Autodesk Inventor part; units mm, degrees
ref_plane "YZ Plane" through (0, 0, 0) normal (1, 0, 0) x (0, 1, 0)
ref_plane "XZ Plane" through (0, 0, 0) normal (0, 1, 0) x (-1, 0, 0)
ref_plane "XY Plane" through (0, 0, 0) normal (0, 0, 1) x (1, 0, 0)
sketch "Szkic1" plane through (0, 0, 0) normal (0, 0, 1) x (1, 0, 0)
  circle A0 centre (0, 0) radius 5.25
  dimension "d0" = 10.5
extrude "Wyciągnięcie proste1" add sketch "Szkic1" along normal blind 5.5
sketch "Szkic2" plane through (0, 0, 5.5) normal (0, 0, 1) x (1, 0, 0)
  circle A0 centre (0, 0) radius 5.25
  circle A1 centre (0, 0) radius 5.85
  dimension "d3" = 11.7
extrude "Wyciągnięcie proste2" add sketch "Szkic2" along normal blind 40 contours A0 | A1
sketch "Szkic3" plane through (0, 0, 45.5) normal (0, 0, 1) x (1, 0, 0)
  circle A0 centre (0, 0) radius 5.85
  circle A1 centre (0, 0) radius 5.55
  dimension "d6" = 11.1
extrude "Wyciągnięcie proste3" add sketch "Szkic3" along normal blind 14.5 contours A1
thread "Gwint1"
sketch "Szkic4" plane through (0, 0, 60) normal (0, 0, 1) x (1, 0, 0)
  circle A0 centre (0, 0) radius 5.25
  dimension "d11" = 10.5
extrude "Wyciągnięcie proste4" add sketch "Szkic4" along normal blind 1
sketch "Szkic5" plane through (0, 0, 61) normal (0, 0, 1) x (1, 0, 0)
  circle A0 centre (0, 0) radius 5.25
  circle A1 centre (-2.2069, 0) radius 2.85
  dimension "d14" = 5.7
extrude "Wyciągnięcie proste5" add sketch "Szkic5" along normal blind 5 contours A1
sketch "Szkic6" plane through (-2.2069, 0, 66) normal (0, 0, 1) x (1, 0, 0)
  circle A0 centre (0, 0) radius 2.85
  circle A1 centre (0, 0) radius 1.8
  point P0 (2.2069, 0)
  dimension "d17" = 3.6
extrude "Wyciągnięcie proste6" add sketch "Szkic6" along normal blind 6 contours A1
properties part number "COTS_GENERIC_Induction_Distance_Sensor"
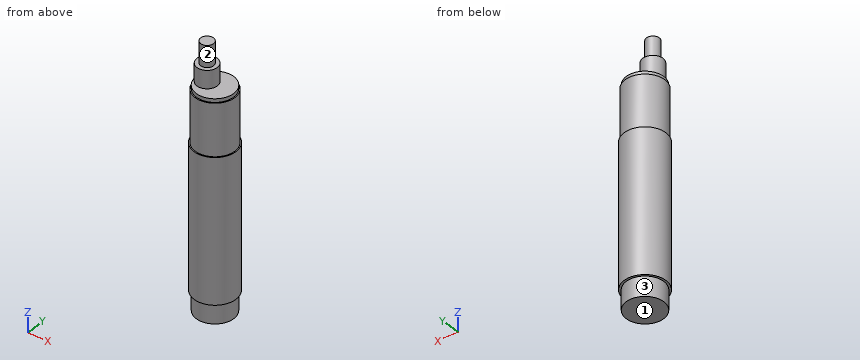
Geometry check sheet. Reference: the model listing, model coordinates, mm. Face numbers are marked on the shaded views. A direction names the side the tool comes from. Round coordinates to 2 decimals unless told otherwise and drop trailing zeros. Order: outer loops, then holes, each group sorted by start corner. A loop starts at its lowest first (then second) coordinate and runs counter-clockwise, first axis right, second up. Notation, with made-up numbers: (-10, 20.25) -> (34, 20.25) arc R21 ccw to (34, 59.25) -> close; hole circle Ø7 at (56.5, 69.25). An arc over 180 degrees is marked (long way). Return JSON: item names as keys, results as strings. Group by question number.
Q1. Section check B-B, the plane x = 4. Record the boundary of the cut face in (y, z), plus the area to 3 significant figures.
Q2. Material ranges on probe 1 along Z at (x, y) = (1.5, 5); probe 2 along Z at (x, y) = (-4, -2); probe 3 along Y at (x, z) = (-0.25, 16.5), recorded low to high. Write a range as from..to.
Q3. Section check D-D, the plane y = 4.5. Record the boundary of the cut face in (x, z).
Q4. Section check A-A, the plane y = 0. Record the boundary of the cut face in (x, z), plus the area to 3 significant figures.
Q5. Gauge pin test, flat ends, axial feed: pin 1 (1 mm diameter, centred on x = -1.5, z = 62.5, fed in from +Y); pin 2 (4 mm diameter, centred on x = 0, z = 54, fed in from +Y); pin 3 (4 mm diameter, centred on x = 4, y = -1.5, fed in from +Z). Record the tip position at first contact, or that the pin passes through.
Q6. Section check C-C, the plane z = 58. Record the boundary of the cut face in (x, y).
Q7. Tool access check on the marked faces 1, 2 and 3. Record the directions out of +Z, -Z, +X, -X, +Y, -Y that give a thin tool (end or side, any length) a straight path to the whole face; none if there is none.
Numbers:
{
 "1": {"outline": "(-4.27, 5.5) -> (-3.4, 5.5) -> (-3.4, 0) -> (3.4, 0) -> (3.4, 5.5) -> (4.27, 5.5) -> (4.27, 45.5) -> (3.85, 45.5) -> (3.85, 60) -> (3.4, 60) -> (3.4, 61) -> (-3.4, 61) -> (-3.4, 60) -> (-3.85, 60) -> (-3.85, 45.5) -> (-4.27, 45.5) -> close", "area": "497 mm^2"},
 "2": {"probe 1": "0..61", "probe 2": "0..66", "probe 3": "-5.84..5.84"},
 "3": {"outline": "(-3.74, 5.5) -> (-2.7, 5.5) -> (-2.7, 0) -> (2.7, 0) -> (2.7, 5.5) -> (3.74, 5.5) -> (3.74, 45.5) -> (3.25, 45.5) -> (3.25, 60) -> (2.7, 60) -> (2.7, 61) -> (-2.7, 61) -> (-2.7, 60) -> (-3.25, 60) -> (-3.25, 45.5) -> (-3.74, 45.5) -> close"},
 "4": {"outline": "(-5.85, 5.5) -> (-5.25, 5.5) -> (-5.25, 0) -> (5.25, 0) -> (5.25, 5.5) -> (5.85, 5.5) -> (5.85, 45.5) -> (5.55, 45.5) -> (5.55, 60) -> (5.25, 60) -> (5.25, 61) -> (0.64, 61) -> (0.64, 66) -> (-0.41, 66) -> (-0.41, 72) -> (-4.01, 72) -> (-4.01, 66) -> (-5.06, 66) -> (-5.06, 61) -> (-5.25, 61) -> (-5.25, 60) -> (-5.55, 60) -> (-5.55, 45.5) -> (-5.85, 45.5) -> close", "area": "747 mm^2"},
 "5": {"pin 1": "y = 2.84", "pin 2": "y = 5.55", "pin 3": "z = 61"},
 "6": {"outline": "circle Ø11.1 at (0, 0)"},
 "7": {"face 1": "-Z, +X, -X, +Y, -Y", "face 2": "+Z", "face 3": "-Z"}
}
